```python
from build123d import *

# Parameters (mm, degrees)
SKETCH1_R                = 410
SKETCH1_R_2              = 360
BOSS_EXTRUDE1_DEPTH      = 80
CUT_EXTRUDE2_DEPTH       = 586.320425066
CUT_EXTRUDE2_DEPTH_BACK  = 586.320425066
SKETCH5_W                = 110
SKETCH5_H                = 80
CUT_EXTRUDE3_DEPTH       = 30
SKETCH6_R                = 31
CUT_EXTRUDE4_DEPTH       = 12
BOSS_EXTRUDE2_REACH      = 926.73
BOSS_EXTRUDE2_END_RADIUS = 410
SKETCH7_W                = 110
SKETCH7_H                = 80
SKETCH9_W                = 110
SKETCH9_H                = 80
CUT_EXTRUDE5_DEPTH       = 41.7
SKETCH10_R               = 31
CUT_EXTRUDE6_DEPTH       = 12


with BuildPart() as part:
    # Sketch1 → Boss-Extrude1 (new body)
    with BuildSketch(Plane(origin=(0, 0, 0), x_dir=(1, 0, 0), z_dir=(0, 1, 0))):
        with Locations(Location((0, 0, 0), (0, 0, 270))):
            Circle(SKETCH1_R)
        with Locations(Location((0, 0, 0), (0, 0, 270))):
            Circle(SKETCH1_R_2, mode=Mode.SUBTRACT)
    extrude(amount=BOSS_EXTRUDE1_DEPTH)

    # Sketch3 → Cut-Extrude2 (cut, two sides: drawn at the far end of the back side and taken through both)
    with BuildSketch(Plane(origin=(0, 80, 0), x_dir=(1, 0, 0), z_dir=(0, 1, 0)).offset(-CUT_EXTRUDE2_DEPTH_BACK)):
        Polygon((-56.5, 287.02643749), (56.5, 287.02643749), (56.5, 362), (33, 362), (33, 370), (-33, 370), (-33, 362), (-56.5, 362), align=None)
    extrude(amount=CUT_EXTRUDE2_DEPTH + CUT_EXTRUDE2_DEPTH_BACK, mode=Mode.SUBTRACT)

    # Sketch5 → Cut-Extrude3 (cut)
    with BuildSketch(Plane.XY.offset(361)):
        with Locations((0, 40)):
            Rectangle(SKETCH5_W, SKETCH5_H)
    extrude(amount=-CUT_EXTRUDE3_DEPTH, mode=Mode.SUBTRACT)

    # Sketch6 → Cut-Extrude4 (cut)
    with BuildSketch(Plane(origin=(0, 0, 361), x_dir=(-1, 0, 0), z_dir=(0, 0, -1))):
        with Locations((0, 40)):
            Circle(SKETCH6_R)
    extrude(amount=-CUT_EXTRUDE4_DEPTH, mode=Mode.SUBTRACT)

    # Boss-Extrude2: up to this cylinder (the profile starts outside it)
    boss_extrude2_end = Plane(origin=(0, 40, 0), z_dir=(0, -1, 0)) * Cylinder(BOSS_EXTRUDE2_END_RADIUS, 2674.46, mode=Mode.PRIVATE)
    # Sketch7 → Boss-Extrude2 (add, up to the surface)
    with BuildSketch(Plane(origin=(415, 0, 0), x_dir=(0, 0, -1), z_dir=(1, 0, 0)), mode=Mode.PRIVATE) as boss_extrude2_sk1:
        with Locations((0, 40)):
            Rectangle(SKETCH7_W, SKETCH7_H)
    boss_extrude2_tool1 = extrude(boss_extrude2_sk1.sketch, amount=-BOSS_EXTRUDE2_REACH, mode=Mode.PRIVATE) - boss_extrude2_end
    add(boss_extrude2_tool1.solids().sort_by_distance((415, 40, 0))[0])

    # Sketch9 → Cut-Extrude5 (cut)
    with BuildSketch(Plane(origin=(-405, 0, 0), x_dir=(0, 0, -1), z_dir=(1, 0, 0))):
        with Locations((0, 40)):
            Rectangle(SKETCH9_W, SKETCH9_H)
    extrude(amount=-CUT_EXTRUDE5_DEPTH, mode=Mode.SUBTRACT)

    # Sketch10 → Cut-Extrude6 (cut)
    with BuildSketch(Plane.ZY.offset(405)):
        with Locations((0, 40)):
            Circle(SKETCH10_R)
    extrude(amount=-CUT_EXTRUDE6_DEPTH, mode=Mode.SUBTRACT)


solid = part.part
```
Geometry check sheet. Reference: the model listing, model coordinates, mm. A direction names the side the tool comes from. Round coordinates to 2 decimals unless told otherwise and drop trailing zeros. Loops run counter-clockwise (first coordinate to the right, second up) from the corner with the lowest first, then second, coordinate; pieces in that order, holes last. Notation, with made-up numbers: (51, -22) -> (92, -22) arc R14 cw to (92, 2) -> close; hole circle Ø7 at (66, 17). An arc over 180 degrees is marked (long way). Use a Markdown table: item, result.
(1) Scan lines: probe 1 along Y at (x, z) = (-402, 0); probe 2 along Z at (x, y) = (-324.5, 49); probe 3 along Z at (x, y) = (130.5, 53.5). Record each from-to range of solid material in increasing order.
Calculated:
| item | result |
|---|---|
| probe 1 | 0 to 9, 71 to 80 |
| probe 2 | -250.6 to -155.88, 155.88 to 250.6 |
| probe 3 | -388.68 to -335.51, 335.51 to 388.68 |
(2) Sectioned sample at C-C (y = 40). Enter the section's corners in (x, z).
Calculated:
| item | result |
|---|---|
| outline | (-406.29, -55) arc R410 ccw to (406.29, -55) -> (415, -55) -> (415, 55) -> (406.29, 55) arc R410 ccw to (-406.29, 55) -> (-405, 55) -> (-405, 31) -> (-393, 31) -> (-393, -31) -> (-405, -31) -> (-405, -55) -> close; hole (-56.5, -362) -> (-33, -362) -> (-33, -370) -> (33, -370) -> (33, -362) -> (56.5, -362) -> (56.5, -355.54) arc R360 ccw to (55, 355.77) -> (55, 361) -> (31, 361) -> (31, 373) -> (-31, 373) -> (-31, 361) -> (-55, 361) -> (-55, 355.77) arc R360 ccw to (-56.5, -355.54) -> close |
(3) Mould release check, pull along Z, two halves, no side actions. Record for faces 1 (the flat face through (-328, 0, 150)), 2 (the cylindrical face through (-8.243, 39.44, 409.917)), 3 (the cylindrical face through (359.913, 39.44, 7.892)): released by +Z, released by -Z, zero draft, split by the parting line, or undercut.
Calculated:
| item | result |
|---|---|
| face 1 | zero draft |
| face 2 | released by +Z |
| face 3 | undercut |
(4) Sectioned sample at D-D (x = -244). Enter the section's corners in (y, z), then the cut area to 3 significant figures.
Calculated:
| item | result |
|---|---|
| outline | (0, -329.49) -> (80, -329.49) -> (80, -264.7) -> (0, -264.7) -> close; (0, 264.7) -> (80, 264.7) -> (80, 329.49) -> (0, 329.49) -> close |
| area | 10,400 mm² |
(5) Sectioned sample at B-B (z = 0). Enter the section's corners in (x, y), then the cut area to 3 significant figures.
Calculated:
| item | result |
|---|---|
| outline | (-405, 0) -> (-360, 0) -> (-360, 80) -> (-405, 80) -> (-405, 71) -> (-393, 71) -> (-393, 9) -> (-405, 9) -> close; (360, 0) -> (415, 0) -> (415, 80) -> (360, 80) -> close |
| area | 7,260 mm² |
(6) Go/stop test with flat-tipped pins: P1, Ø1.5, axis at x = 254, y = 43, coming from the +Z side; P2, Ø2.5, axis at x = 412, y = 32, coming from the -Z side; P3, Ø1.5, axis at y = 45.5, z = -273.5, coming from the +X side. Record where each tip stops, or that it passes through.
Calculated:
| item | result |
|---|---|
| P1 | z = 322.44 |
| P2 | z = -55 |
| P3 | x = 306.12 |
(7) Set-up check for faces 4 (the cylindrical face through (4.036, 70.736, 366.916)), 5 (the flat face through (-405, 58.34, 25.21)), 6 (the cylindrical face through (-399.084, 70.736, -4.036)), 7 (the cylindrical face through (8.243, 39.44, -409.917)), 8 (the flat face through (-25.21, 58.34, 361)): record each of +Z, -Z, +X, -X, +Y, -Y from which the full face is reachable in a straight line by a thin tool's end or side.
Calculated:
| item | result |
|---|---|
| face 4 | none |
| face 5 | -X, +Y, -Y |
| face 6 | -X |
| face 7 | -Z, +Y, -Y |
| face 8 | +Y, -Y |
(8) Sectioned sample at A-A (x = 0). Enter the section's corners in (y, z), then the cut area to 3 significant figures.
Calculated:
| item | result |
|---|---|
| outline | (0, -410) -> (80, -410) -> (80, -370) -> (0, -370) -> close; (0, 361) -> (9, 361) -> (9, 373) -> (71, 373) -> (71, 361) -> (80, 361) -> (80, 410) -> (0, 410) -> close |
| area | 6,380 mm² |
